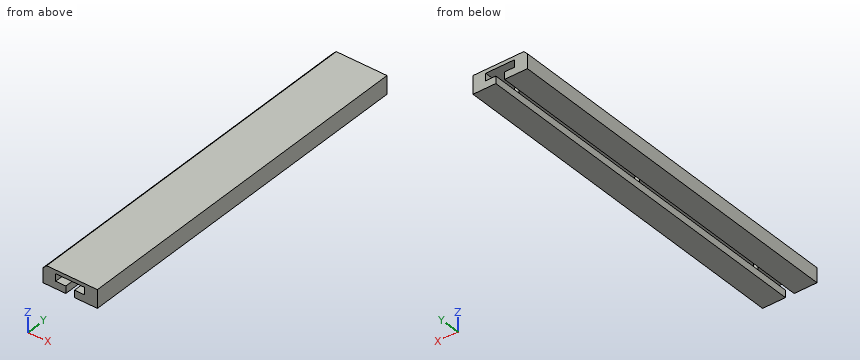
from build123d import *

# Parameters (mm, degrees)
F0_W     = 15
F0_H     = 5
F1_DEPTH = 100
F2_W     = 1.2
F2_H     = 2
F3_DEPTH = 113.7
F4_R     = 0.5
F5_DEPTH = 2.87
F6_SIZE  = 1


with BuildPart() as f1:
    # F0 (on Front) → F1 (new body)
    with BuildSketch(Plane.XZ):
        with Locations((0, 2.5)):
            Rectangle(F0_W, F0_H)
    extrude(amount=F1_DEPTH)

    # F2 (on face) → F3 (cut)
    with BuildSketch(Plane(origin=(0, 0, 0), x_dir=(-1, 0, 0), z_dir=(0, 1, 0))):
        Polygon((-4, 2), (-1.2, 2), (0, 2), (0, 4), (-4, 4), align=None)
        with Locations((-0.6, 1)):
            Rectangle(F2_W, F2_H)
        with Locations((0.6, 1)):
            Rectangle(F2_W, F2_H)
        Polygon((0, 4), (0, 2), (1.2, 2), (4, 2), (4, 4), align=None)
    extrude(amount=-F3_DEPTH, mode=Mode.SUBTRACT)

    # F4 (on face) → F5 (join)
    with BuildSketch(Plane.XY.offset(2)):
        with Locations((-2.2, -8.50577)):
            Circle(F4_R)
        with Locations((-2.2, -50)):
            Circle(F4_R)
        with Locations((-2.2, -90.948157)):
            Circle(F4_R)
        with Locations((2.2, -90.948157)):
            Circle(F4_R)
        with Locations((2.2, -50)):
            Circle(F4_R)
        with Locations((2.2, -8.50577)):
            Circle(F4_R)
    extrude(amount=F5_DEPTH)

    # F6
    f6_edges = [f1.edges().sort_by_distance(p)[0] for p in [
        (-7.5, -50, 5),
    ]]
    chamfer(f6_edges, length=F6_SIZE)


solid = f1.part
Design review of the part built by this model. Coordinates are the model's own, in mm. Round coordinates to 2 decimals unless told otherwise and drop trailing zeros. Write each loop counter-clockwise with the first axis right and the second up, starting at its lowest first coordinate (ties: lowest second). Pieces come first, ordered by that corner, then holes.
Item 1: Consider section A-A on y = -62. Give the boundary of the cut face in (x, z).
Item 2: Consider section B-B on z = 3.05. Give the boundary of the cut face in (x, y).
Item 3: Wall thickness on L1, parallel to Z at x = 3.75, y = -48; L2, parallel to X at y = -46, z = 1.6; L3, parallel to X at y = -38, z = 3.55: over which ranges is each line inside the solid? List them lowest first.
Check values:
1. outline: (-7.5, 0) - (-1.2, 0) - (-1.2, 2) - (-4, 2) - (-4, 4) - (4, 4) - (4, 2) - (1.2, 2) - (1.2, 0) - (7.5, 0) - (7.5, 5) - (-6.5, 5) - (-7.5, 4) - close
2. outline: (-7.5, -100) - (-4, -100) - (-4, 0) - (-7.5, 0) - close; circle Ø1 at (-2.2, -90.95); circle Ø1 at (-2.2, -50); circle Ø1 at (-2.2, -8.51); circle Ø1 at (2.2, -90.95); circle Ø1 at (2.2, -50); circle Ø1 at (2.2, -8.51); (4, -100) - (7.5, -100) - (7.5, 0) - (4, 0) - close
3. L1: z = 0 to 2, 4 to 5
3. L2: x = -7.5 to -1.2, 1.2 to 7.5
3. L3: x = -7.5 to -4, 4 to 7.5
